```python
from build123d import *

# Parameters (mm, degrees)
SKETCH1_W           = 150
SKETCH1_H           = 120
BOSS_EXTRUDE1_DEPTH = 30
CHAMFER1_SIZE       = 20


with BuildPart() as part:
    # Sketch1 → Boss-Extrude1 (new body, symmetric)
    with BuildSketch(Plane.XY):
        with Locations((75, 60)):
            Rectangle(SKETCH1_W, SKETCH1_H)
    extrude(amount=BOSS_EXTRUDE1_DEPTH, both=True)

    # Chamfer1
    chamfer1_edges = [part.edges().sort_by_distance(p)[0] for p in [
        (0, 120, 0),
        (150, 120, 0),
        (150, 0, 0),
        (0, 0, 0),
    ]]
    chamfer(chamfer1_edges, length=CHAMFER1_SIZE)


solid = part.part
```
The model under review builds one solid part; all positions refer to its coordinate system, in mm. Coordinates: 2 decimals unless noted, no trailing zeros. Loops run counter-clockwise (first coordinate to the right, second up) from the corner with the lowest first, then second, coordinate; pieces in that order, holes last. Notation, with made-up numbers: (59, 36) -> (72, 36) arc R17 ccw to (72, 63) -> close; hole circle Ø5 at (39, -3). An arc over 180 degrees is marked (long way). Answer as CSV lines item,"result".
Item 1: Take a section at C-C, the plane x = 139.5. State the section outline as (y, z) points.
Results below:
outline,"(9.5, -30) -> (110.5, -30) -> (110.5, 30) -> (9.5, 30) -> close"
Item 2: Take a section at B-B, the plane y = 109.5. State the section outline as (x, z) points, and give its area (3 significant figures).
Results below:
outline,"(9.5, -30) -> (140.5, -30) -> (140.5, 30) -> (9.5, 30) -> close"
area,"7,860 mm2"
Item 3: Take a section at A-A, the plane z = -23. State the section outline as (x, y) points.
Results below:
outline,"(0, 20) -> (20, 0) -> (130, 0) -> (150, 20) -> (150, 100) -> (130, 120) -> (20, 120) -> (0, 100) -> close"
Item 4: For L1, parallel to Y at x = 137, z = 22; L2, parallel to Y at x = 6, z = 22; L3, parallel to X at y = 115, z = 2.5, list the stretches that pass through material, from the lowest coordinate up.
Results below:
L1,"y = 7 to 113"
L2,"y = 14 to 106"
L3,"x = 15 to 135"
